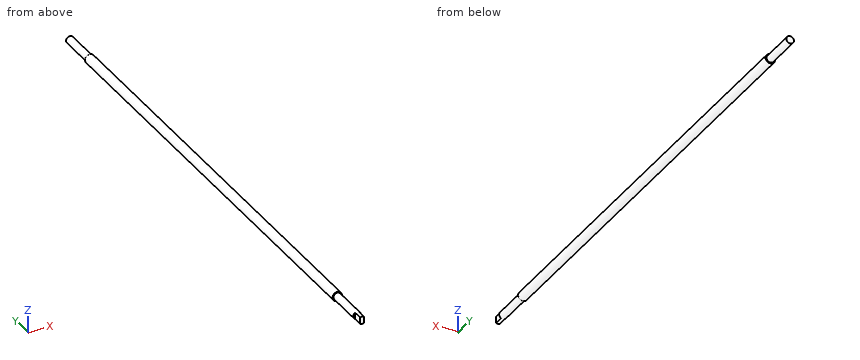
from build123d import *

# Parameters (mm, degrees)
F0_R     = 5
F1_DEPTH = 295
F2_R     = 9
F2_R_2   = 4
F3_DEPTH = 50
F4_R     = 5
F4_R_2   = 4
F5_DEPTH = 40
F7_DEPTH = 10


with BuildPart() as f1:
    # F0 (on Front) → F1 (new body, symmetric)
    with BuildSketch(Plane.XZ):
        Circle(F0_R)
    extrude(amount=F1_DEPTH, both=True)

    # F2 (on face) → F3 (cut)
    with BuildSketch(Plane.XZ.offset(295)):
        Circle(F2_R)
        Circle(F2_R_2, mode=Mode.SUBTRACT)
    extrude(amount=-F3_DEPTH, mode=Mode.SUBTRACT)

    # F4 (on face) → F5 (cut)
    with BuildSketch(Plane(origin=(0, 295, 0), x_dir=(-1, 0, 0), z_dir=(0, 1, 0))):
        Circle(F4_R)
        Circle(F4_R_2, mode=Mode.SUBTRACT)
    extrude(amount=-F5_DEPTH, mode=Mode.SUBTRACT)

    # F6 (on face) → F7 (cut)
    with BuildSketch(Plane.XZ.offset(295)):
        Polygon((2, 9.214783), (2, -9.214783), (-2, -9.214783), (-2, 9.214783), (-11.609545, 9.214783), (-11.609545, -12.255539), (8.235434, -15.570633), (8.235434, 9.214783), align=None)
    extrude(amount=-F7_DEPTH, mode=Mode.SUBTRACT)


solid = f1.part
Model file for the job. Use its own axes, mm. Give positions to 0.01 mm unless a question says otherwise; leave off trailing zeros. Write each loop counter-clockwise with the first axis right and the second up, starting at its lowest first coordinate (ties: lowest second). Pieces come first, ordered by that corner, then holes. Notation, with made-up numbers: M -25,77.5 L 11,77.5 A22 cw 11,86.5 Z; hole C -7.5,88 d5. An arc over 180 degrees is marked long. One line per item, written item: value. Start each with the question number.
Q1. Drop flat-ended pins along their axis: pin 1 Ø3.5 at (y, z) = (-292.5, 0) entering from +X; pin 2 Ø5.5 at (y, z) = (-288, 1.5) entering from -X; pin 3 Ø2 at (y, z) = (48.5, -4) entering from -X; pin 4 Ø3 at (x, y) = (1.5, 9.5) entering from -Z. Give the stop position or say it passes through.
Q2. Saw through at A-A, the plane z = 0. Write the cut outline in (x, y).
Q3. Saw through at C-C, the plane y = 137. Write the cut outline in (x, z).
Q4. Saw through at B-B, the plane x = 0. Write the cut outline in (y, z), plus the area to 3 significant figures.
Q5. Probe probe 1 along Y at (x, z) = (-2.5, -4); probe 2 along X at (y, z) = (-99, 1); probe 3 along Y at (x, z) = (-2.75, 1). List the from-to ranges inside material, lowest first. Write a range as [from, to].
Output values:
1. pin 1: stops at x = 2
1. pin 2: stops at x = -2
1. pin 3: stops at x = -4
1. pin 4: stops at z = -5
2. outline: M -5,-245 L -4,-245 L -4,-285 L -2,-285 L -2,-295 L 2,-295 L 2,-285 L 4,-285 L 4,-245 L 5,-245 L 5,255 L 4,255 L 4,295 L -4,295 L -4,255 L -5,255 Z
3. outline: C 0,0 d10
4. outline: M -295,-4 L -245,-4 L -245,-5 L 255,-5 L 255,-4 L 295,-4 L 295,4 L 255,4 L 255,5 L -245,5 L -245,4 L -295,4 Z
4. area: 5,720 mm²
5. probe 1: y = [-245, 255]
5. probe 2: x = [-4.9, 4.9]
5. probe 3: y = [-285, 295]
